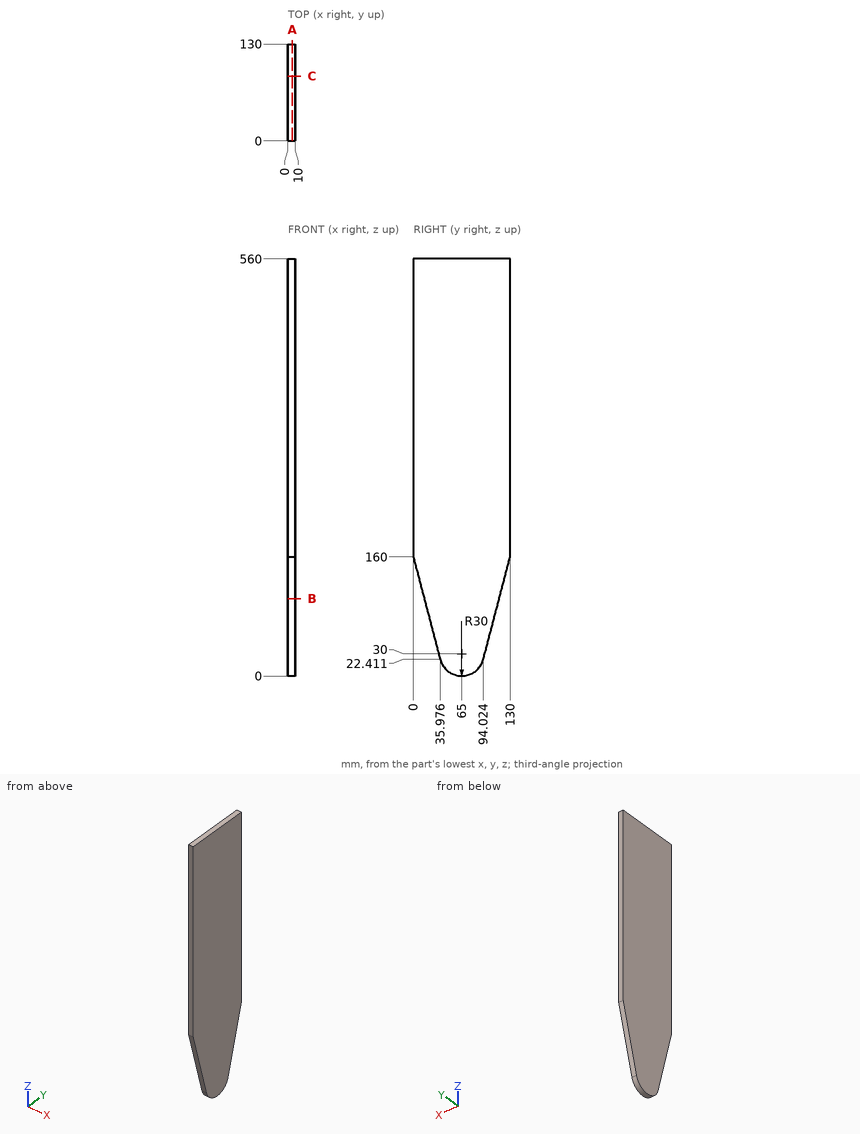
Input: dimensioned drawing with shaded views. Units: mm. Origin: part minimum x, y, z. Round coordinates to 2 decimals unless told otherwise and drop trailing zeros. Order: outer loops, then holes, each group sorted by start corner. A loop starts at its lowest first (then second) coordinate and runs counter-clockwise, first axis right, second up. Notation, with made-up numbers: (27.5, 45.25) - (84.5, 45.25) arc R27 ccw to (84.5, 72.25) - close; hole circle Ø8 at (61.5, -39). An arc over 180 degrees is marked (long way). Write item = value, one per line. Start each with the question number.
Q1. Cut plane B-B on z = 104. Return the cut outline in (x, y), and give its area (3 significant figures).
Q2. Ray query, line 1 (Z direction, x = 1.25, y = 65.5); line 2 (Z direction, x = 8.25, y = 77) (1 decimal); line 3 (Y direction, x = 5.75, z = 31). Return the intervals inside material, ascending. Write a range as from..to.
Q3. Cut plane C-C on y = 87. Return the cut outline in (x, z).
Q4. Cut plane A-A on x = 6. Return the cut outline in (y, z), and give its area (3 significant figures).
Q5. Pin query (flat end, axial travel): pin 1 (2 mm diameter, centred on y = 13.5, z = 429, fed in from -X). Return the tip coordinate at first contact, or that it passes through.
Outcome:
q1.outline = (0, 14.64) - (10, 14.64) - (10, 115.36) - (0, 115.36) - close
q1.area = 1,010 mm^2
q2.line_1 = 0..560
q2.line_2 = 2.5..560
q2.line_3 = 33.73..96.27
q3.outline = (0, 9.6) - (10, 9.6) - (10, 560) - (0, 560) - close
q4.outline = (0, 160) - (35.98, 22.41) arc R30 ccw to (94.02, 22.41) - (130, 160) - (130, 560) - (0, 560) - close
q4.area = 65,900 mm^2
q5.pin_1 = 0
